from build123d import *

# Parameters (mm, degrees)
BOSS_EXTRUDE1_DEPTH                       = 3.175
SKETCH3_W                                 = 12.7
SKETCH3_H                                 = 19.05
BOSS_EXTRUDE2_DEPTH                       = 5.08
CUT_EXTRUDE2_DEPTH                        = 27.096877687
CUT_EXTRUDE3_DEPTH                        = 27.096877687
F_2_56_TAPPED_HOLE1_D                     = 1.778
SKETCH9_W                                 = 22.225
SKETCH9_H                                 = 5.08
BOSS_EXTRUDE3_DEPTH                       = 5.08
SKETCH12_R                                = 1.5875
CUT_EXTRUDE4_DEPTH                        = 3.302
SKETCH13_W                                = 4.826
SKETCH13_H                                = 6.35
SKETCH13_W_2                              = 5.08
BOSS_EXTRUDE4_DEPTH                       = 5.08
F_1_16_0_0625_DIAMETER_HOLE1_D            = 1.5875
F_3_64_0_04688_DIAMETER_HOLE1_D           = 1.190752
F_3_64_0_04688_DIAMETER_HOLE1_ON_FACE_2_D = 1.190752


with BuildPart() as part:
    # Sketch1 → Boss-Extrude1 (new body)
    with BuildSketch(Plane.XY):
        with BuildLine():
            Line((9.271, 5.08), (12.7, 5.08))
            Line((12.7, 5.08), (12.7, 0))
            Line((12.7, 0), (0, 0))
            Line((0, 0), (0, 5.08))
            Line((0, 5.08), (3.429, 5.08))
            ThreePointArc((3.429, 5.08), (6.35, 2.159), (9.271, 5.08))
        make_face()
    extrude(amount=BOSS_EXTRUDE1_DEPTH)

    # Sketch3 → Boss-Extrude2 (add)
    with BuildSketch(Plane.XZ):
        with Locations((6.35, 12.7)):
            Rectangle(SKETCH3_W, SKETCH3_H)
    extrude(amount=-BOSS_EXTRUDE2_DEPTH)

    # Sketch7 → Cut-Extrude2 (cut, through all)
    with BuildSketch(Plane(origin=(0, 5.08, 0), x_dir=(1, 0, 0), z_dir=(0, 1, 0))):
        with BuildLine():
            Line((2.54, -3.175), (10.16, -3.175))
            ThreePointArc((10.16, -3.175), (11.176, -4.191), (10.16, -5.207))
            Line((10.16, -5.207), (2.54, -5.207))
            ThreePointArc((2.54, -5.207), (1.524, -4.191), (2.54, -3.175))
        make_face()
    extrude(amount=-CUT_EXTRUDE2_DEPTH, mode=Mode.SUBTRACT)

    # Sketch6 → Cut-Extrude3 (cut, through all)
    with BuildSketch(Plane.XY.offset(22.225)):
        Polygon((6.173223305, 5.08), (6.35, 4.903223305), (6.526776695, 5.08), align=None)
    extrude(amount=-CUT_EXTRUDE3_DEPTH, mode=Mode.SUBTRACT)

    # #2-56 Tapped Hole1 (through all)
    with Locations(Plane(origin=(11.176, 5.08, 1.5875), x_dir=(0, 0, 1), z_dir=(0, 1, 0))):
        with Locations((0, 0), (0, -9.652)):
            Hole(F_2_56_TAPPED_HOLE1_D / 2)

    # Sketch9 → Boss-Extrude3 (add)
    with BuildSketch(Plane.ZY):
        with Locations((11.1125, 2.54)):
            Rectangle(SKETCH9_W, SKETCH9_H)
    extrude(amount=BOSS_EXTRUDE3_DEPTH)

    # Sketch12 → Cut-Extrude4 (cut)
    with BuildSketch(Plane(origin=(0, 5.08, 0), x_dir=(1, 0, 0), z_dir=(0, 1, 0))):
        with Locations(Location((10.16, -17.145, 0), (0, 0, 270))):
            Circle(SKETCH12_R)
        with Locations(Location((10.16, -9.525, 0), (0, 0, 270))):
            Circle(SKETCH12_R)
    extrude(amount=-CUT_EXTRUDE4_DEPTH, mode=Mode.SUBTRACT)

    # Sketch13 → Boss-Extrude4 (add)
    with BuildSketch(Plane(origin=(0, 5.08, 0), x_dir=(1, 0, 0), z_dir=(0, 1, 0))):
        with Locations((-2.667, -3.175)):
            Rectangle(SKETCH13_W, SKETCH13_H)
        with Locations((-2.54, -19.05)):
            Rectangle(SKETCH13_W_2, SKETCH13_H)
    extrude(amount=BOSS_EXTRUDE4_DEPTH)

    # 1/16 (0.0625) Diameter Hole1 (through all)
    with Locations(Plane.XY.offset(22.225)):
        with Locations((-2.54, 7.62)):
            Hole(F_1_16_0_0625_DIAMETER_HOLE1_D / 2)

    # 3/64 (0.04688) Diameter Hole1 (through all)
    with Locations(Plane(origin=(10.16, 5.08, 17.145), x_dir=(0, 0, 1), z_dir=(0, 1, 0))):
        with Locations((0, 0)):
            Hole(F_3_64_0_04688_DIAMETER_HOLE1_D / 2)

    # 3/64 (0.04688) Diameter Hole1 on face 2 (through all)
    with Locations(Plane(origin=(10.16, 1.778, 9.525), x_dir=(0, 0, 1), z_dir=(0, 1, 0))):
        with Locations((0, 0)):
            Hole(F_3_64_0_04688_DIAMETER_HOLE1_ON_FACE_2_D / 2)


solid = part.part
Design review of the part built by this model. Coordinates are the model's own, in mm. A direction names the side the tool comes from. Coordinates: 2 decimals unless noted, no trailing zeros. Loops run counter-clockwise (first coordinate to the right, second up) from the corner with the lowest first, then second, coordinate; pieces in that order, holes last. Notation, with made-up numbers: (39.25, 84) - (84.25, 84) arc R6 cw to (84.25, 93) - close; hole circle Ø2 at (88, 61). An arc over 180 degrees is marked (long way). Use CSV: the item, a comma, the result in double quotes. Start each with the question number.
1. Add section C-C on x = 4. Give the boundary of the cut face in (y, z) (3 decimals), plus the area to 3 significant figures.
2. For faces 4 (the cylindrical face through (10.23, 3.45, 7.94)), 5 (the cylindrical face through (6.29, 2.16, 1.57)), 6 (the flat face through (6, 2, 3.175)), 7 (the flat face through (-4, 8, 15.875)), list the 3-axis set-ups (+Z, -Z, +X, -X, +Y, -Y) from which the entire face can be reached by the end or side of a thin tool; tool diameter is ignored.
3. Add section A-A on x = -2.54. Give the boundary of the cut face in (y, z) (3 decimals), plus the area to 3 significant figures.
4. Add section D-D on z = 7. Give the boundary of the cut face in (x, y).
5. Add section B-B on y = 7.62. Give the boundary of the cut face in (x, z) (3 decimals), plus the area to 3 significant figures.
6. Clearance check with flat-ended pins moving along their axes: pin 1 (1.9 mm diameter, centred on x = 10.16, z = 17.145, fed in from +Y); pin 2 (1.5 mm diameter, centred on y = 6.5, z = 19, fed in from +X); pin 3 (4 mm diameter, centred on x = 6.5, y = 5, fed in from -Z). State where each tip first meets the part, or that it passes through.
7. To check wall thickness, follow probe 1 along Z at (x, y) = (8.25, 1.25) (3 decimals); probe 2 along Z at (x, y) = (-2.5, 6) (3 decimals); probe 3 along X at (y, z) = (1.5, 2). State the ranges of each line that lie inside material, in increasing order.
8. Mouldability with a two-part tool opening along X and no side actions: class faces 1 (the flat face through (10, 5.08, 14)), 2 (the cylindrical face through (-2.91, 6.92, 3.13)), 3 (the flat face through (12.7, 3, 11)) as released by +X, released by -X, zero draft, split by the parting line, or undercut.
Resolved:
1,outline,"(0, 0) - (3.345, 0) - (3.345, 3.175) - (0, 3.175) - close; (0, 5.207) - (5.08, 5.207) - (5.08, 22.225) - (0, 22.225) - close"
1,area,"97.1 mm2"
2,face 4,"+Y"
2,face 5,"-Z, +Y"
2,face 6,"+Y, -Y"
2,face 7,"+X, -X, +Y"
3,outline,"(0, 0) - (6.826, 0) - (6.826, 6.35) - (5.08, 6.35) - (5.08, 15.875) - (6.826, 15.875) - (6.826, 22.225) - (0, 22.225) - close; (8.414, 0) - (10.16, 0) - (10.16, 6.35) - (8.414, 6.35) - close; (8.414, 15.875) - (10.16, 15.875) - (10.16, 22.225) - (8.414, 22.225) - close"
3,area,"157 mm2"
4,outline,"(-5.08, 0) - (12.7, 0) - (12.7, 5.08) - (6.53, 5.08) - (6.35, 4.9) - (6.17, 5.08) - (-5.08, 5.08) - close"
5,outline,"(-5.08, 0) - (-3.334, 0) - (-3.334, 6.35) - (-5.08, 6.35) - close; (-5.08, 15.875) - (-3.334, 15.875) - (-3.334, 22.225) - (-5.08, 22.225) - close; (-1.746, 0) - (-0.254, 0) - (-0.254, 6.35) - (-1.746, 6.35) - close; (-1.746, 15.875) - (0, 15.875) - (0, 22.225) - (-1.746, 22.225) - close"
5,area,"42.7 mm2"
6,pin 1,"y = 1.78"
6,pin 2,"x = 0"
6,pin 3,"z = 5.21"
7,probe 1,"0 to 3.175, 5.207 to 22.225"
7,probe 2,"0 to 6.35, 15.875 to 22.225"
7,probe 3,"-5.08 to 0.74, 2.31 to 10.39, 11.96 to 12.7"
8,face 1,"zero draft"
8,face 2,"undercut"
8,face 3,"released by +X"
